The listing builds one solid part. Answer for the finished solid, in the listing's coordinates (mm). Face numbers are marked on the shaded views. A direction names the side the tool comes from. Give positions to 0.01 mm unless a question says otherwise; leave off trailing zeros. Loops run counter-clockwise (first coordinate to the right, second up) from the corner with the lowest first, then second, coordinate; pieces in that order, holes last. Notation, with made-up numbers: (-34, -16) - (11, -16) arc R19 cw to (11, 20) - close; hole circle Ø6 at (16, -11.75). An arc over 180 degrees is marked (long way). Write item = value, one per line. Start each with the question number.
1) Flat-ended cylindrical pins translate along their axes: P1, Ø1, axis at x = 77, y = 10.5, coming from the -Z side; P2, Ø2, axis at y = -21, z = 144.5, coming from the +X side; P3, Ø4, axis at x = 36.5, z = 31, coming from the +Y side. Find the tip coordinate at first contact, or state that the pin passes through.
2) Which of the six approach directions +Z, -Z, +X, -X, +Y, -Y give full straight-line access (tool end or side, diameter ignored) to the marked faces 1, 2 and 3?
3) The mould has two halves that part along X. Classify the marked faces 4, 5, 6 and 7: +X half, -X half, draft (parallel to the pull), parting line (faces both ways), or undercut.
4) Consider probe 1 along X at (y, z) = (-96, -16); probe 2 along Y at (x, z) = (28, 74). Determine where each line is inside the solid, lowest interval first.
5) The part is cut by section A-A on y = -78. Write down the section's boundary in (x, z), plus the area to 3 significant figures.
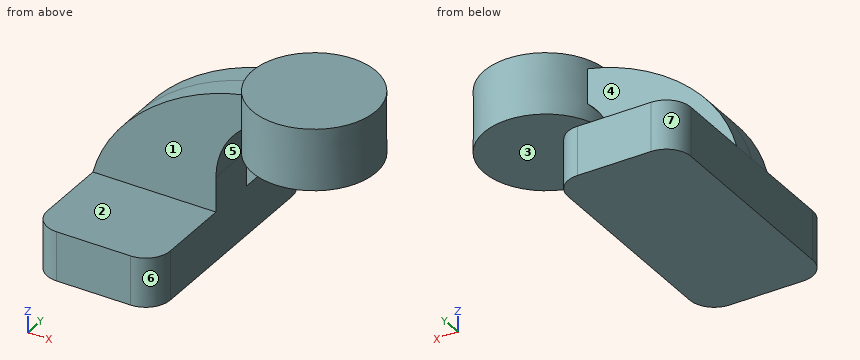
from build123d import *

# Parameters (mm, degrees)
F1_DEPTH = 127
F2_DEPTH = 25.4
F4_R     = 25.4


with BuildPart() as f1:
    # F0 (on Front) → F1 (new body, symmetric)
    with BuildSketch(Plane.XZ):
        Polygon((42.44389, 25.4), (-63.5, 25.4), (-63.5, -25.4), (63.5, -25.4), (63.5, 25.4), align=None)
    extrude(amount=F1_DEPTH, both=True)

    # F0 (on Front) → F2 (join, symmetric)
    with BuildSketch(Plane.XZ):
        with BuildLine():
            add(Edge.make_bspline(
                [(-63.5, 25.4), (-42.358271, 108.126874), (62.167687, 166.074246), (139.7, 158.507851)],
                knots=[0, 0, 0, 0, 242.9155, 242.9155, 242.9155, 242.9155], degree=3))
            Line((-63.5, 25.4), (42.44389, 25.4))
            Line((42.44389, 25.4), (42.44389, 61.251742))
            ThreePointArc((42.44389, 61.251742), (70.929545, 130.022196), (139.7, 158.507851))
        make_face()
        with BuildLine():
            Line((42.44389, 61.251742), (42.44389, 25.4))
            Line((42.44389, 25.4), (63.5, 25.4))
            Line((63.5, 25.4), (63.5, 61.251742))
            ThreePointArc((63.5, 61.251742), (85.818463, 115.133278), (139.7, 137.451742))
            Line((139.7, 137.451742), (149.225, 137.451742))
            Line((149.225, 137.451742), (149.225, 158.507851))
            Line((149.225, 158.507851), (139.7, 158.507851))
            ThreePointArc((139.7, 158.507851), (70.929545, 130.022196), (42.44389, 61.251742))
        make_face()
    extrude(amount=F2_DEPTH, both=True)

    # F0 (on Front) → F3 (revolve)
    with BuildSketch(Plane.XZ):
        Polygon((149.225, 165.1), (149.225, 158.507851), (149.225, 137.451742), (149.225, 101.6), (213.216364, 101.6), (213.1069, 165.1), align=None)
    revolve(axis=Axis((149.225, 0, 133.35), (0, 0, -1)))

    # F4
    f4_edges = [f1.edges().sort_by_distance(p)[0] for p in [
        (63.5, -127, 0),
        (-63.5, -127, 0),
        (63.5, 127, 0),
        (-63.5, 127, 0),
    ]]
    fillet(f4_edges, radius=F4_R)


solid = f1.part
Answer below:
q1.P1 = 103.82
q1.P2 = 209.93
q1.P3 = 25.4
q2.face_1 = +Z, -X, -Y
q2.face_2 = +Z, +X, -X, -Y
q2.face_3 = -Z, +X, +Y, -Y
q3.face_4 = draft
q3.face_5 = undercut
q3.face_6 = +X half
q3.face_7 = -X half
q4.probe_1 = -63.5 to 63.5
q4.probe_2 = -25.4 to 25.4
q5.outline = (-63.5, -25.4) - (63.5, -25.4) - (63.5, 25.4) - (-63.5, 25.4) - close
q5.area = 6,450 mm2
